```python
from build123d import *

# Parameters (mm, degrees)
BOSS_EXTRUDE1_DEPTH     = 10
CUT_EXTRUDE1_DEPTH      = 104.60672567
CUT_EXTRUDE1_DEPTH_BACK = 104.60672567
SKETCH2_R               = 2
CUT_EXTRUDE2_DEPTH      = 106.044531529
CUT_EXTRUDE2_DEPTH_BACK = 106.044531529
SKETCH3_R               = 2


with BuildPart() as part:
    # Sketch1 → Boss-Extrude1 (new, symmetric)
    with BuildSketch(Plane.XY):
        Polygon((99.852319163, 10), (-50.147680837, 25.76563529), (-50.147680837, 0), (99.852319163, 0), align=None)
    extrude(amount=BOSS_EXTRUDE1_DEPTH, both=True)

    # Sketch2 → Cut-Extrude1 (cut, two sides: drawn at the far end of the back side and taken through both)
    with BuildSketch(Plane.XZ.offset(-CUT_EXTRUDE1_DEPTH_BACK)):
        Circle(SKETCH2_R)
    extrude(amount=CUT_EXTRUDE1_DEPTH + CUT_EXTRUDE1_DEPTH_BACK, mode=Mode.SUBTRACT)

    # Sketch3 → Cut-Extrude2 (cut, two sides: drawn at the far end of the back side and taken through both)
    with BuildSketch(Plane(origin=(0, 0, -10), x_dir=(-1, 0, 0), z_dir=(0, 0, -1)).offset(-CUT_EXTRUDE2_DEPTH_BACK)):
        with Locations((24.103932874, 18.000785679)):
            Circle(SKETCH3_R)
        with Locations((-41.8489822, 11.068854977)):
            Circle(SKETCH3_R)
    extrude(amount=CUT_EXTRUDE2_DEPTH + CUT_EXTRUDE2_DEPTH_BACK, mode=Mode.SUBTRACT)


solid = part.part
```
Geometry check sheet. Reference: the model listing, model coordinates, mm. Coordinates: 2 decimals unless noted, no trailing zeros. Order: outer loops, then holes, each group sorted by start corner. A loop starts at its lowest first (then second) coordinate and runs counter-clockwise, first axis right, second up.
Q1. Depth check by flat-ended pin: pin 1 Ø2.5 at (x, z) = (0, 0) entering from -Y. Enter the tip coordinate at first touch or a pass-through.
Reply:
pin 1: passes through
Q2. Thickness scan on probe 1 along Z at (x, y) = (0, 13.5); probe 2 along X at (y, z) = (9.25, -2.5); probe 3 along Y at (x, z) = (43, -4). Record the ranges inside material, lowest first.
Reply:
probe 1: z = -10 to -2, 2 to 10
probe 2: x = -50.15 to 41.02, 42.68 to 99.85
probe 3: y = 0 to 9.43, 12.7 to 15.98
Q3. Draft check along X on faces 1 (the face through (24, 0, 0)), 2 (the face through (43.847, 11.157, 0.14)), 3 (the face through (-50.148, 13, 0)), 4 (the face through (25.902, 17.772, 0.14)). Enter one of: released by +X, released by -X, zero draft, split by the parting line, or undercut.
Reply:
face 1: zero draft
face 2: undercut
face 3: released by -X
face 4: released by +X
Q4. Sectioned sample at C-C on z = 5.5. Record the cut outline in (x, y).
Reply:
outline: (-50.15, 0) - (99.85, 0) - (99.85, 10) - (-50.15, 25.77) - close; hole circle Ø4 at (-24.1, 18); hole circle Ø4 at (41.85, 11.07)
Q5. Sectioned sample at A-A on z = 0. Record the cut outline in (x, y).
Reply:
outline: (-50.15, 0) - (-2, 0) - (-2, 20.71) - (-50.15, 25.77) - close; (2, 0) - (99.85, 0) - (99.85, 10) - (2, 20.28) - close; hole circle Ø4 at (-24.1, 18); hole circle Ø4 at (41.85, 11.07)
Q6. Sectioned sample at B-B on x = 0. Record the cut outline in (y, z).
Reply:
outline: (0, -10) - (20.49, -10) - (20.49, -2) - (0, -2) - close; (0, 2) - (20.49, 2) - (20.49, 10) - (0, 10) - close
Q7. Sectioned sample at D-D on x = 22. Record the cut outline in (y, z).
Reply:
outline: (0, -10) - (18.18, -10) - (18.18, 10) - (0, 10) - close
